Work out the finished part from the listing and answer in its coordinate system (mm). A direction names the side the tool comes from. Coordinates: 2 decimals unless noted, no trailing zeros. Order: outer loops, then holes, each group sorted by start corner. A loop starts at its lowest first (then second) coordinate and runs counter-clockwise, first axis right, second up. Notation, with made-up numbers: M 86.5,64 L 124.5,64 A20 cw 124.5,102 Z; hole C -20.5,37 d7. An arc over 180 degrees is marked long. Answer in a Markdown table with one row per item. Add a question column.
Item 1: The mould has two halves that part along Z. Classify faces 1 (the face through (-11, 23, -118.5)), 2 (the face through (-30, 0, 0)), 3 (the face through (3, 74, 2)), 4 (the face through (0, 49, 138.5)): released by +Z, released by -Z, zero draft, split by the parting line, or undercut.
Item 2: The part is cut by section B-B (x = -14). Write down the section's boundary in (y, z), then the cut area to 3 significant figures.
Item 3: The part is cut by section A-A (x = -30). Write down the section's boundary in (y, z), then the cut area to 3 significant figures.
Item 4: The part is cut by section C-C (y = 15). State how many separate pieces and enclosed holes the cut face has, then the cut area to 3 significant figures.
Item 5: Consider line 1 (Z direction, x = -10.5, y = 35); line 2 (X direction, y = 49, z = -33.5); line 3 (Y direction, x = -58.5, z = -4.5). Determine where each line is inside the solid, lowest interval first. Write a range as from..to.
Item 6: Which of the six approach directions +Z, -Z, +X, -X, +Y, -Y give full straight-line access (tool end or side, diameter ignored) to faces 5 (the face through (-23, 3, -98)), 6 (the face through (0, 35, -35)), 7 (the face through (-13.14, 33.09, -98.22)), 8 (the face through (-13.14, 33.09, 98.78))?
Item 7: Flat-ended cylindrical pins translate along their axes: pin 1 Ø11 at (x, y) = (9, 14.5) entering from -Z; pin 2 Ø8 at (x, y) = (10, 34) entering from +Z; pin 3 Ø3 at (x, z) = (-0.5, -40) entering from -Y. Find the tip coordinate at first contact, or state that the pin passes through.
Item 8: The part is cut by section D-D (z = -0.5). Write down the section's boundary in (x, y), then the cut area to 3 significant figures.
from build123d import *
from OCP.BRepFilletAPI import BRepFilletAPI_MakeChamfer

# Parameters (mm, degrees)
SKETCH_1_W          = 6
SKETCH_1_H          = 277
EXTRUDE_1_DEPTH     = 150
SKETCH_2_W          = 20
SKETCH_2_H          = 40
SKETCH_2_W_2        = 60
SKETCH_2_H_2        = 20
EXTRUDE_2_DEPTH     = 6
EXTRUDE_3_DEPTH     = 7
CHAMFER_2_SIZE      = 54.949548389
CHAMFER_2_SIZE_2    = 20
SKETCH_5_W          = 10
SKETCH_5_H          = 30
EXTRUDE_4_DEPTH     = 10
CHAMFER_3_SIZE      = 17.320508076
CHAMFER_3_SIZE_2    = 10
SKETCH_6_W          = 30
SKETCH_6_H          = 35
CUT_EXTRUDE_1_DEPTH = 10
FILLET_2_R          = 50


with BuildPart() as part:
    # Эскиз1 → Бобышка-Вытянуть1 (new body)
    with BuildSketch(Plane(origin=(0, 0, 0), x_dir=(1, 0, 0), z_dir=(0, 1, 0))):
        Rectangle(SKETCH_1_W, SKETCH_1_H)
    extrude(amount=EXTRUDE_1_DEPTH)

    # Эскиз2 → Бобышка-Вытянуть2 (add)
    with BuildSketch(Plane(origin=(0, 0, 0), x_dir=(1, 0, 0), z_dir=(0, 1, 0))):
        with Locations((-13, 98.5)):
            Rectangle(SKETCH_2_W, SKETCH_2_H)
        with Locations((-13, -98.5)):
            Rectangle(SKETCH_2_W, SKETCH_2_H)
        with Locations((-33, 0)):
            Rectangle(SKETCH_2_W_2, SKETCH_2_H_2)
    extrude(amount=EXTRUDE_2_DEPTH)

    # Эскиз3 → Бобышка-Вытянуть3 (add)
    with BuildSketch(Plane.XY.offset(3.5)):
        Polygon((-3, 6), (-51, 6), (-3, 150), align=None)
    extrude(amount=-EXTRUDE_3_DEPTH)

    # Фаска2
    chamfer_2_edges_1 = [part.edges().sort_by_distance(p)[0] for p in [
        (-3, 6, 98.5),
    ]]
    chamfer_2_side_1 = [part.faces().sort_by_distance(p)[0] for p in [
        (-3, 6.4, 98.5),
    ]]
    chamfer_2_edges_2 = [part.edges().sort_by_distance(p)[0] for p in [
        (-3, 6, -98.5),
    ]]
    chamfer_2_side_2 = [part.faces().sort_by_distance(p)[0] for p in [
        (-3, 6.4, -98.5),
    ]]
    chamfer_2 = BRepFilletAPI_MakeChamfer(part.part.solid().wrapped)
    for e in chamfer_2_edges_1:
        chamfer_2.Add(CHAMFER_2_SIZE - 0.0001, CHAMFER_2_SIZE_2 - 0.0001, e.wrapped, chamfer_2_side_1[0].wrapped)
    for e in chamfer_2_edges_2:
        chamfer_2.Add(CHAMFER_2_SIZE - 0.0001, CHAMFER_2_SIZE_2 - 0.0001, e.wrapped, chamfer_2_side_2[0].wrapped)
    add(Compound.cast(chamfer_2.Shape()), mode=Mode.REPLACE)  # a hair under: the kernel refuses the full size

    # Эскиз5 → Бобышка-Вытянуть4 (add)
    with BuildSketch(Plane(origin=(3, 0, 0), x_dir=(0, 0, -1), z_dir=(1, 0, 0))):
        with Locations((-108.5, 35)):
            Rectangle(SKETCH_5_W, SKETCH_5_H)
        with Locations((108.5, 35)):
            Rectangle(SKETCH_5_W, SKETCH_5_H)
    extrude(amount=EXTRUDE_4_DEPTH)

    # Фаска3
    chamfer_3_edges_1 = [part.edges().sort_by_distance(p)[0] for p in [
        (3, 20, 108.5),
    ]]
    chamfer_3_side_1 = [part.faces().sort_by_distance(p)[0] for p in [
        (3, 19.8, 108.5),
    ]]
    chamfer_3_edges_2 = [part.edges().sort_by_distance(p)[0] for p in [
        (3, 20, -108.5),
    ]]
    chamfer_3_side_2 = [part.faces().sort_by_distance(p)[0] for p in [
        (3, 19.8, -108.5),
    ]]
    chamfer_3 = BRepFilletAPI_MakeChamfer(part.part.solid().wrapped)
    for e in chamfer_3_edges_1:
        chamfer_3.Add(CHAMFER_3_SIZE - 0.0001, CHAMFER_3_SIZE_2 - 0.0001, e.wrapped, chamfer_3_side_1[0].wrapped)
    for e in chamfer_3_edges_2:
        chamfer_3.Add(CHAMFER_3_SIZE - 0.0001, CHAMFER_3_SIZE_2 - 0.0001, e.wrapped, chamfer_3_side_2[0].wrapped)
    add(Compound.cast(chamfer_3.Shape()), mode=Mode.REPLACE)  # a hair under: the kernel refuses the full size

    # Эскиз6 → Вырез-Вытянуть1 (cut)
    with BuildSketch(Plane(origin=(3, 0, 0), x_dir=(0, 0, -1), z_dir=(1, 0, 0))):
        with Locations((-35, 17.5)):
            Rectangle(SKETCH_6_W, SKETCH_6_H)
        with Locations((35, 17.5)):
            Rectangle(SKETCH_6_W, SKETCH_6_H)
    extrude(amount=-CUT_EXTRUDE_1_DEPTH, mode=Mode.SUBTRACT)

    # Скругление2
    fillet_2_edges = [part.edges().sort_by_distance(p)[0] for p in [
        (0, 150, 138.5),
        (0, 150, -138.5),
    ]]
    fillet(fillet_2_edges, radius=FILLET_2_R)


solid = part.part
Reply:
| question | item | result |
|---|---|---|
| 1 | face 1 | released by -Z |
| 1 | face 2 | zero draft |
| 1 | face 3 | undercut |
| 1 | face 4 | released by +Z |
| 2 | outline | M 0,-118.5 L 30.73,-118.5 L 30.73,-78.5 L 0,-78.5 Z; M 0,-10 L 6,-10 L 6,-3.5 L 117,-3.5 L 117,3.5 L 6,3.5 L 6,10 L 0,10 Z; M 0,78.5 L 30.73,78.5 L 30.73,118.5 L 0,118.5 Z |
| 2 | area | 3,360 mm2 |
| 3 | outline | M 0,-10 L 6,-10 L 6,-3.5 L 69,-3.5 L 69,3.5 L 6,3.5 L 6,10 L 0,10 Z |
| 3 | area | 561 mm2 |
| 4 | separate pieces | 3 |
| 4 | enclosed holes | 0 |
| 4 | area | 3,100 mm2 |
| 5 | line 1 | z = -118.5..-78.5, -3.5..3.5, 78.5..118.5 |
| 5 | line 2 | x = -3..3 |
| 5 | line 3 | y = 0..6 |
| 6 | face 5 | -Z, -X, +Y, -Y |
| 6 | face 6 | +X, -X, -Y |
| 6 | face 7 | -Z, -X, +Y |
| 6 | face 8 | +Z, -X, +Y |
| 7 | pin 1 | stops at z = -113.5 |
| 7 | pin 2 | stops at z = 113.5 |
| 7 | pin 3 | stops at y = 35 |
| 8 | outline | M -63,0 L 3,0 L 3,150 L -3,150 L -51,6 L -63,6 Z |
| 8 | area | 4,720 mm2 |
